Model file for the job. Use its own axes, mm. A direction names the side the tool comes from. Round coordinates to 2 decimals unless told otherwise and drop trailing zeros. Loops run counter-clockwise (first coordinate to the right, second up) from the corner with the lowest first, then second, coordinate; pieces in that order, holes last.
Autodesk Inventor part; units mm, degrees
ref_plane "YZ Plane" through (0, 0, 0) normal (1, 0, 0) x (0, 1, 0)
ref_plane "XZ Plane" through (0, 0, 0) normal (0, 1, 0) x (-1, 0, 0)
ref_plane "XY Plane" through (0, 0, 0) normal (0, 0, 1) x (1, 0, 0)
sketch "Sketch1" plane through (0, 0, 0) normal (0, 0, 1) x (1, 0, 0)
  circle A0 centre (0, 0) radius 10
  line L0 (10, 0) -> (10, -38)
  line L1 (10, -38) -> (-10, -38)
  line L2 (-10, -38) -> (-10, 0)
  circle A1 centre (0, 6) radius 2.1
  circle A2 centre (-6, 0) radius 2.1
  circle A3 centre (6, 0) radius 2.1
  circle A4 centre (0, -6) radius 2.1
  circle A5 centre (0, -22) radius 2.1
  circle A6 centre (0, -34) radius 2.1
  line L3 (10, -18) -> (24, -18)
  line L4 (24, -18) -> (24, -38)
  line L5 (24, -38) -> (10, -38)
  line L6 (10, -38) -> (10, -18)
  circle A7 centre (18, -22) radius 2.1
  circle A8 centre (18, -34) radius 2.1
  line L7 (-10, 0) -> (-8.1, 0)
  line L8 (-3.9, 0) -> (3.9, 0)
  line L9 (8.1, 0) -> (10, 0)
  dimension "d0" = 20
  dimension "d1" = 38
  dimension "d2" = 4.2
  dimension "d3" = 4.2
  dimension "d4" = 4.2
  dimension "d5" = 4.2
  dimension "d6" = 4.2
  dimension "d7" = 4.2
  dimension "d8" = 14
  dimension "d9" = 4.2
  dimension "d10" = 4.2
extrude "Extrusion1" add sketch "Sketch1" along normal blind 3 contours L9 A3 L8 A2 L7 A0 | L0 L1 L2 A0 | A0 L7 A2 L8 A3 L9 | L3 L4 L5 L0
sketch "Sketch2" plane through (0, 0, 3) normal (0, 0, 1) x (1, 0, 0)
  circle A0 centre (0, 6) radius 2.6
  circle A1 centre (-6, 0) radius 2.6
  circle A2 centre (6, 0) radius 2.6
  circle A3 centre (0, -6) radius 2.6
  circle A4 centre (0, -22) radius 2.6
  circle A5 centre (0, -34) radius 2.6
  circle A6 centre (18, -22) radius 2.6
  circle A7 centre (18, -34) radius 2.6
  point P0 (0, 0)
  dimension "d13" = 5.2
  dimension "d14" = 5.2
  dimension "d15" = 5.2
  dimension "d16" = 5.2
  dimension "d17" = 5.2
  dimension "d18" = 5.2
  dimension "d19" = 5.2
  dimension "d20" = 5.2
extrude "Extrusion2" cut sketch "Sketch2" against normal blind 1
properties part number "Wheel_holder"
Q1. Slice it at D-D on y = 6. Give the cut face in (x, z), plus the area to 3 significant figures.
Q2. Tool access for faces 1 (the face through (10, -9, 1)), 2 (the face through (-0.338, -31.422, 2.507)), 3 (the face through (24, -28, 1)): list every direction of +Z, -Z, +X, -X, +Y, -Y with a clear straight run to the whole face (end or side of a thin tool).
Q3. Slice it at C-C on x = 6. Give the cut face in (y, z).
Q4. Flat gauge pins, fed straight in: P1, Ø1.5, axis at x = 1.5, y = -21, coming from the +Z side; P2, Ø1.5, axis at x = 16.5, z = 1.5, coming from the +Y side. Where does each tip first touch, or does it go through?
Q5. Probe line 1 (X direction, y = -22, z = 1.05); line 2 (Y direction, x = 18, z = 1.1); line 3 (Y direction, x = 0, z = 2.7). List the from-to ranges inside material, lowest first.
Q6. Slice it at B-B on y = -34. Give the cut face in (x, z), plus the area to 3 significant figures.
Q7. Slice it at A-A on z = 1.05. State how many separate pieces and enclosed holes the cut face has, plus the area to 3 significant figures.
Q8. Pull direction X, two halves, no side cores. Call faces 4 (the face through (-0.338, -19.422, 2.507)), 5 (the face through (1.13, -23.77, 0.99)), 6 (the face through (3, -19, 0)), 7 (the face through (-10, -19, 1)): pulls with the +X half, pulls with the -X half, needs draft (parallel to the pull), parting line crosses it, or undercut.
Reply:
1. outline: (-8, 0) - (-2.1, 0) - (-2.1, 2) - (-2.6, 2) - (-2.6, 3) - (-8, 3) - close; (2.1, 0) - (8, 0) - (8, 3) - (2.6, 3) - (2.6, 2) - (2.1, 2) - close
1. area: 34.4 mm2
2. face 1: +Z, -Z, +X, +Y
2. face 2: +Z
2. face 3: +Z, -Z, +X, +Y, -Y
3. outline: (-38, 0) - (-2.1, 0) - (-2.1, 2) - (-2.6, 2) - (-2.6, 3) - (-38, 3) - close; (2.1, 0) - (8, 0) - (8, 3) - (2.6, 3) - (2.6, 2) - (2.1, 2) - close
4. P1: stops at z = 2
4. P2: stops at y = -18
5. line 1: x = -10 to -2.1, 2.1 to 15.9, 20.1 to 24
5. line 2: y = -38 to -36.1, -31.9 to -24.1, -19.9 to -18
5. line 3: y = -38 to -36.6, -31.4 to -24.6, -19.4 to -8.6, -3.4 to 3.4, 8.6 to 10
6. outline: (-10, 0) - (-2.1, 0) - (-2.1, 2) - (-2.6, 2) - (-2.6, 3) - (-10, 3) - close; (2.1, 0) - (15.9, 0) - (15.9, 2) - (15.4, 2) - (15.4, 3) - (2.6, 3) - (2.6, 2) - (2.1, 2) - close; (20.1, 0) - (24, 0) - (24, 3) - (20.6, 3) - (20.6, 2) - (20.1, 2) - close
6. area: 74.8 mm2
7. separate pieces: 1
7. enclosed holes: 8
7. area: 1,090 mm2
8. face 4: undercut
8. face 5: undercut
8. face 6: needs draft
8. face 7: pulls with the -X half
